Can you work these out from the model? Positions are in its coordinate system, mm. A direction names the side the tool comes from. Give positions to 0.01 mm unless a question says otherwise; leave off trailing zeros. Loops run counter-clockwise (first coordinate to the right, second up) from the corner with the lowest first, then second, coordinate; pieces in that order, holes last. Notation, with made-up numbers: (80, 52.25) - (116, 52.25) arc R9 cw to (116, 64.25) - close; hole circle Ø10 at (41.5, 14). An arc over 180 degrees is marked (long way). Answer as a JSON object with one key per item and string values. Group by question number.
Item 1: Thinking about a two-plate mould opening in X: for faces 1 (the cylindrical face through (-64.8, -3.6, -2.3)), 2 (the conical face through (-69.997, -4.667, -4.941)), 3 (the flat face through (-10, -2, 53)), which applies, pulls with the +X half, pulls with the -X half, needs draft (parallel to the pull), parting line crosses it, or undercut?
Item 2: Suppose I cut it at A-A on z = 22. Write out the boundary of the cut face in (x, y).
Item 3: Which directions (+Z, -Z, +X, -X, +Y, -Y) give clear straight access to the entire face, cutting with the end or side of a thin tool? Please do faces 4 (the flat face through (-21, -2, -7)), 5 (the cylindrical face through (29.88, -4.89, -3.28)), 6 (the cylindrical face through (-71, -2, 35)), 7 (the flat face through (31.1, 0, 45)), 8 (the flat face through (5.75, -2, 52)).
Item 4: Please list where these lines run through material, in increasing order: L1, parallel to Z at x = 27.4, y = -1.95; L2, parallel to X at y = -1.85, z = 48.4; L3, parallel to X at y = -3.1, z = 48.4.
Item 5: Suppose I cut it at B-B on z = 40.5. Write out the boundary of the cut face in (x, y).
Item 6: Will these pins go through, and if not, where does the flat tip stop? pin 1 (3 mm diameter, centred on x = -68, z = 47.5, fed in from +Y); pin 2 (4 mm diameter, centred on x = 27.4, z = 48.4, fed in from -Y); pin 3 (8.5 mm diameter, centred on x = -67.4, z = -2.5, fed in from -Y); pin 4 (2 mm diameter, centred on y = -2, z = 52, fed in from -X).
from build123d import *

# Parameters (mm, degrees)
CYLINDER001_R           = 2
CYLINDER001_DEPTH       = 10
SKETCH037_W             = 7.5
SKETCH037_H             = 7.5
EXTRUDE045_DEPTH        = 10
BOX089_W                = 11
BOX089_H                = 10
BOX089_DEPTH            = 35
BODY005_PLACEMENT_ANGLE = 90
BODY006_PLACEMENT_ANGLE = 90
CYLINDER003_R           = 2
CYLINDER003_DEPTH       = 10
CYLINDER002_R           = 1.7
CYLINDER002_DEPTH       = 10
SKETCH032_R             = 2.6
EXTRUDE043_DEPTH        = 0.8
EXTRUDE040_DEPTH        = 3
EXTRUDE038_DEPTH        = 2
EXTRUDE041_DEPTH        = 0.8


with BuildPart() as battery_cable:
    # Cylinder001 → Cylinder001 (new body)
    with BuildSketch(Plane(origin=(-66.5, 0, 35), x_dir=(0, 0, 1), z_dir=(-1, 0, 0))):
        Circle(CYLINDER001_R)
    extrude(amount=CYLINDER001_DEPTH)


with BuildPart() as switch_hole002:
    # Sketch037 → Extrude045 (new body)
    with BuildSketch(Plane.YZ.offset(35)):
        with Locations((0, 38.5)):
            Rectangle(SKETCH037_W, SKETCH037_H)
    extrude(amount=EXTRUDE045_DEPTH)


with BuildPart() as switch_hole002_1:
    # Extrude045 placement: moved
    add(switch_hole002.part.moved(Location((-9.5, 0, 0))))


with BuildPart() as dips001:
    # Box089 → Box089 (new body)
    with BuildSketch(Plane(origin=(-15, 0.5, 13.5), x_dir=(0, 0, -1), z_dir=(1, 0, 0))):
        with Locations((5.5, 5)):
            Rectangle(BOX089_W, BOX089_H)
    extrude(amount=BOX089_DEPTH)


with BuildPart() as switch_hole001:
    # Body005 base: copy of switch hole002
    add(switch_hole002_1.part)


with BuildPart() as switch_hole001_1:
    # Body005 placement: moved
    add(switch_hole001.part.moved(Location((40.5, 0, 22))).rotate(Axis((40.5, 0, 22), (0, -1, 0)), BODY005_PLACEMENT_ANGLE))


with BuildPart() as switch_hole:
    # Body006 base: copy of switch hole002
    add(switch_hole002_1.part)


with BuildPart() as switch_hole_1:
    # Body006 placement: moved
    add(switch_hole.part.moved(Location((16, 0, 22))).rotate(Axis((16, 0, 22), (0, -1, 0)), BODY006_PLACEMENT_ANGLE))


with BuildPart() as cable:
    # Cylinder003 → Cylinder003 (new body)
    with BuildSketch(Plane(origin=(-65.5, 0, 12), x_dir=(0, -1, 0), z_dir=(-1, 0, 0))):
        Circle(CYLINDER003_R)
    extrude(amount=CYLINDER003_DEPTH)


with BuildPart() as common_sub:
    # Cylinder002 → Cylinder002 (new body)
    with BuildSketch(Plane(origin=(25, -1.5, 28), x_dir=(1, 0, 0), z_dir=(0, 1, 0))):
        Circle(CYLINDER002_R)
    extrude(amount=CYLINDER002_DEPTH)

    # Fusion033: union battery cable, switch hole002, dips001, switch hole001, switch hole, cable
    add(battery_cable.part)
    add(switch_hole002_1.part)
    add(dips001.part)
    add(switch_hole001_1.part)
    add(switch_hole_1.part)
    add(cable.part)


with BuildPart() as sweep_body:
    # Sweep: sweep along a path in Sketch034
    with BuildLine(Plane.XZ.offset(10)) as sweep_path:
        Line((32, 12), (32, 48.4))
        ThreePointArc((32, 48.4), (30.652691, 51.652691), (27.4, 53))
        Line((27.4, 53), (-20, 53))
    # Sketch033 → Sweep (sweep)
    with BuildSketch(Plane.YZ):
        Polygon((-5.3, 51.4), (-3.7, 53), (-3.7, 54), (-6, 54), (-6, 51.4), align=None)
    sweep(path=sweep_path.line)


with BuildPart() as fusion:
    # Sketch032 → Extrude043 (new body)
    with BuildSketch(Plane.XZ.offset(10)):
        with Locations((27.4, 48.5)):
            Circle(SKETCH032_R)
    extrude(amount=EXTRUDE043_DEPTH)


with BuildPart() as fusion_1:
    # Extrude043 placement: moved
    add(fusion.part.moved(Location((0, 5.5, 0))))

    # Fusion: union Sweep body
    add(sweep_body.part)


with BuildPart() as bottom003:
    # Sketch028 → Extrude040 (new body)
    with BuildSketch(Plane.XZ.offset(10)):
        with BuildLine():
            ThreePointArc((32, 48.4), (30.652691, 51.652691), (27.4, 53))
            Line((27.4, 53), (-20, 53))
            Line((-20, 53), (-20, 51))
            Line((-20, 51), (27.4, 51))
            ThreePointArc((30, 48.4), (29.238478, 50.238478), (27.4, 51))
            Line((30, 23), (30, 48.4))
            Line((32, 23), (30, 23))
            Line((32, 48.4), (32, 23))
        make_face()
    extrude(amount=EXTRUDE040_DEPTH)


with BuildPart() as bottom003_1:
    # Extrude040 placement: moved
    add(bottom003.part.moved(Location((0, 8.5, 0))))


with BuildPart() as bottom004:
    # Sketch030 → Extrude038 (new body)
    with BuildSketch(Plane.XZ.offset(10)):
        with BuildLine():
            ThreePointArc((32, 48.4), (30.652691, 51.652691), (27.4, 53))
            Line((27.4, 53), (-20, 53))
            Line((-20, 53), (-20, 52.1))
            Line((-20, 52.1), (27.4, 52.1))
            ThreePointArc((31.1, 48.4), (30.016295, 51.016295), (27.4, 52.1))
            Line((31.1, 23), (31.1, 48.4))
            Line((32, 23), (31.1, 23))
            Line((32, 48.4), (32, 23))
        make_face()
    extrude(amount=EXTRUDE038_DEPTH)


with BuildPart() as bottom004_1:
    # Extrude038 placement: moved
    add(bottom004.part.moved(Location((0, 10.5, 0))))


with BuildPart() as screw_hole_bottom002:
    # Sketch003 → Revolve (revolve)
    with BuildSketch(Plane.XY):
        Polygon((1.6, 3), (1.6, 2), (0, 2), (0, 1.8), (2.6, 1.8), (2.6, 0), (4.6, 0), (4.6, 3), align=None)
    revolve(axis=Axis((0, 0, 0), (0, 1, 0)))


with BuildPart() as screw_hole_bottom002_1:
    # Body003 placement: moved
    add(screw_hole_bottom002.part.moved(Location((27.4, -4.5, 48.4))))


with BuildPart() as bottom:
    # Sketch031 → Extrude041 (new body)
    with BuildSketch(Plane.XZ.offset(10)):
        with BuildLine():
            ThreePointArc((32, 48.4), (30.652691, 51.652691), (27.4, 53))
            Line((27.4, 53), (-20, 53))
            Line((-20, 53), (-20, 23))
            Line((-20, 23), (32, 23))
            Line((32, 48.4), (32, 23))
        make_face()
    extrude(amount=EXTRUDE041_DEPTH)


with BuildPart() as bottom_1:
    # Extrude041 placement: moved
    add(bottom.part.moved(Location((0, 5.5, 0))))

    # Fusion029: union bottom003, bottom004, screw hole bottom002
    add(bottom003_1.part)
    add(bottom004_1.part)
    add(screw_hole_bottom002_1.part)

    # Cut: cut Fusion
    add(fusion_1.part, mode=Mode.SUBTRACT)


with BuildPart() as part_mirroring005:
    # Part__Mirroring005: instance of bottom
    add(bottom_1.part.mirror(Plane(origin=(-20, 0, 0), x_dir=(0, -1, 0), z_dir=(1, 0, 0))))


with BuildPart() as part_mirroring006:
    # Part__Mirroring006: instance of Part__Mirroring005
    add(part_mirroring005.part.mirror(Plane(origin=(0, 0, 23), x_dir=(0, 1, 0), z_dir=(0, 0, 1))))


with BuildPart() as bottom007:
    # Part__Mirroring004: instance of bottom
    add(bottom_1.part.mirror(Plane(origin=(0, 0, 23), x_dir=(0, 1, 0), z_dir=(0, 0, 1))))

    # Fusion031: union bottom, Part__Mirroring006, Part__Mirroring005
    add(bottom_1.part)
    add(part_mirroring006.part)
    add(part_mirroring005.part)

    # Cut026: cut common sub
    add(common_sub.part, mode=Mode.SUBTRACT)


solid = bottom007.part
Worked out:
{
 "1": {"face 1": "undercut", "face 2": "pulls with the -X half", "face 3": "needs draft"},
 "2": {"outline": "(-72, -3.7) - (-70.4, -5.3) - (30.4, -5.3) - (32, -3.7) - (32, 0.5) - (31.1, 0.5) - (31.1, -1.5) - (30, -1.5) - (30, -4.5) - (-70, -4.5) - (-70, -1.5) - (-71.1, -1.5) - (-71.1, 0.5) - (-72, 0.5) - close"},
 "3": {"face 4": "-Z, +X, -X, +Y, -Y", "face 5": "-Y", "face 6": "-X", "face 7": "+Y", "face 8": "+Z, +Y"},
 "4": {"L1": "z = -7 to -4, -0.8 to 2.2, 43.8 to 46.8, 50 to 53", "L2": "x = -72 to -69, -65.8 to -62.8, 22.8 to 25.8, 29 to 32", "L3": "x = -72 to -70, -64.8 to -62.8, 22.8 to 24.8, 30 to 32"},
 "5": {"outline": "(-72, -3.7) - (-70.4, -5.3) - (30.4, -5.3) - (31.95, -3.75) - (30, -3.75) - (30, -4.5) - (-70, -4.5) - (-70, -1.5) - (-71.1, -1.5) - (-71.1, 0.5) - (-72, 0.5) - close"},
 "6": {"pin 1": "stops at y = -1.5", "pin 2": "stops at y = -2.7", "pin 3": "stops at y = -5.3", "pin 4": "stops at x = -71.19"}
}
